Model file for the job. Use its own axes, mm. Give positions to 0.01 mm unless a question says otherwise; leave off trailing zeros. Order: outer loops, then holes, each group sorted by start corner. A loop starts at its lowest first (then second) coordinate and runs counter-clockwise, first axis right, second up. Notation, with made-up numbers: (40, -7.75) -> (70, -7.75) arc R20 ccw to (70, 24.25) -> close; hole circle Ø1 at (64.5, 18). An arc over 180 degrees is marked (long way). Use CSV: the item, a comma, the result in double quotes. Start each with the question number.
1. Cut at A-A on y = 92.5. List the corners of the cut face in (x, z).
2. Wall check: line 1 (Z direction, x = 8.5, y = 61); line 2 (X direction, y = -66.5, z = 1.75); line 3 (X direction, y = -39, z = 2). Give the ranges that are in metal, low to high. Write a range as from..to.
3. Cut at B-B on x = 42.5. List the corners of the cut face in (y, z), then the cut area to 3 significant figures.
4. Cut at D-D on y = -54. List the corners of the cut face in (x, z), then the cut area to 3 significant figures.
5. Drop flat-ended pins along their axis: pin 1 (4.5 mm diameter, centred on x = -48.94, y = -85.6, fed in from -Z); pin 2 (4.5 mm diameter, centred on x = 48.94, y = -85.6, fed in from +Z); pin 3 (8 mm diameter, centred on x = -41, z = -6, fed in from -Y). Give the stop position or say it passes through.
6. Cut at C-C on x = -9. List the corners of the cut face in (y, z).
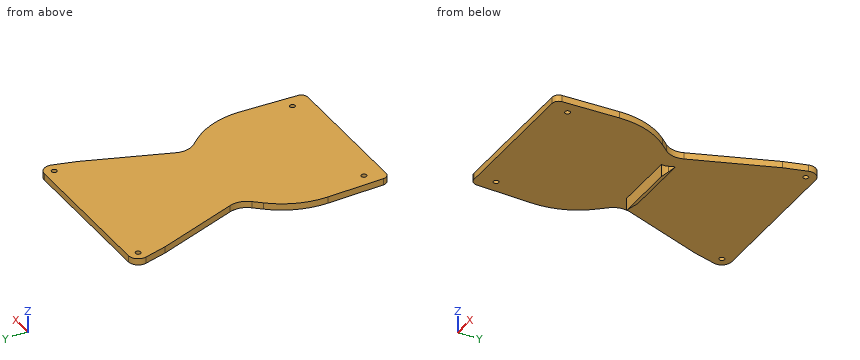
```python
from build123d import *

# Parameters (mm, degrees)
SKETCH1_R           = 2
BOSS_EXTRUDE1_DEPTH = 5
BOSS_EXTRUDE2_DEPTH = 10
CHAMFER2_SIZE       = 10


with BuildPart() as part:
    # Sketch1 → Boss-Extrude1 (new body)
    with BuildSketch(Plane.XY):
        with BuildLine():
            Line((-39.95406266, -4.540740277), (-45.172708428, -10.510426525))
            ThreePointArc((-45.172708428, -10.510426525), (-56.503917554, -29.818144261), (-59.968772691, -51.935536587))
            Line((-59.968772691, -51.935536587), (-58.57362931, -95.161294716))
            ThreePointArc((-58.57362931, -95.161294716), (-57.054271725, -98.592107569), (-53.576231585, -100))
            Line((-53.576231585, -100), (-50, -100))
            Line((-50, -100), (50, -100))
            Line((50, -100), (53.576231585, -100))
            ThreePointArc((53.576231585, -100), (57.054271725, -98.592107569), (58.57362931, -95.161294716))
            Line((58.57362931, -95.161294716), (59.968772691, -51.935536587))
            ThreePointArc((59.968772691, -51.935536587), (56.503917554, -29.818144261), (45.172708428, -10.510426525))
            Line((45.172708428, -10.510426525), (39.95406266, -4.540740277))
            ThreePointArc((39.95406266, -4.540740277), (36.502239109, 2.577573283), (37.151850455, 10.461955241))
            Line((37.151850455, 10.461955241), (60, 73.236730193))
            Line((60, 73.236730193), (64.733567494, 90.51871221))
            ThreePointArc((64.733567494, 90.51871221), (63.462787034, 97.049194521), (57.5, 100))
            Line((57.5, 100), (55, 100))
            Line((55, 100), (-55, 100))
            Line((-55, 100), (-57.5, 100))
            ThreePointArc((-57.5, 100), (-63.462787034, 97.049194521), (-64.733567494, 90.51871221))
            Line((-64.733567494, 90.51871221), (-60, 73.236730193))
            Line((-60, 73.236730193), (-37.151850455, 10.461955241))
            ThreePointArc((-37.151850455, 10.461955241), (-36.502239109, 2.577573283), (-39.95406266, -4.540740277))
        make_face()
        with Locations((-57.5, 92.5)):
            Circle(SKETCH1_R, mode=Mode.SUBTRACT)
        with Locations((57.5, 92.5)):
            Circle(SKETCH1_R, mode=Mode.SUBTRACT)
        with Locations((48.939097244, -85.598196118)):
            Circle(SKETCH1_R, mode=Mode.SUBTRACT)
        with Locations((-48.939097244, -85.598196118)):
            Circle(SKETCH1_R, mode=Mode.SUBTRACT)
    extrude(amount=BOSS_EXTRUDE1_DEPTH)

    # Sketch2 → Boss-Extrude2 (add)
    with BuildSketch(Plane(origin=(0, 0, 0), x_dir=(-1, 0, 0), z_dir=(0, 0, -1))):
        with BuildLine():
            Line((-23.747944524, 0.5), (23.747944524, 0.5))
            ThreePointArc((23.747944524, 0.5), (23.669056818, 3.144030102), (24.253462846, 5.723872742))
            Line((24.253462846, 5.723872742), (25.870507592, 10.166666667))
            Line((25.870507592, 10.166666667), (-25.870507592, 10.166666667))
            Line((-25.870507592, 10.166666667), (-24.253462846, 5.723872742))
            ThreePointArc((-24.253462846, 5.723872742), (-23.669056818, 3.144030102), (-23.747944524, 0.5))
        make_face()
    extrude(amount=BOSS_EXTRUDE2_DEPTH)

    # Chamfer2
    # the kernel refuses this chamfer: 10 mm, written as the material it takes off along each edge
    with BuildSketch(Plane(origin=(-51.587337472, 10.166666667, -10), x_dir=(0, 0.027495876610586317, 0.9996219169112968), z_dir=(1, 0, 0))) as chamfer2_piece_1_section:
        Polygon((CHAMFER2_SIZE * 0.999621916911, CHAMFER2_SIZE * 0.0274958766106), (-CHAMFER2_SIZE * 0.0274958766106, CHAMFER2_SIZE * 0.999621916911), (0, 0), align=None)
    chamfer2_piece_1 = extrude(amount=103.174674944, mode=Mode.PRIVATE)
    chamfer2_piece_1 = split(chamfer2_piece_1, bisect_by=Plane(origin=(0, 6.862625123, 0), z_dir=(0, 0, -1)), keep=Keep.TOP, mode=Mode.PRIVATE)
    add(chamfer2_piece_1, mode=Mode.SUBTRACT)


solid = part.part
```
Verdict:
1,outline,"(-65, 0) -> (-59.5, 0) -> (-59.5, 5) -> (-65, 5) -> close; (-55.5, 0) -> (55.5, 0) -> (55.5, 5) -> (-55.5, 5) -> close; (59.5, 0) -> (65, 0) -> (65, 5) -> (59.5, 5) -> close"
2,line 1,"0..5"
2,line 2,"-59.5..59.5"
2,line 3,"-58.98..58.98"
3,outline,"(-100, 0) -> (-7.45, 0) -> (-7.45, 5) -> (-100, 5) -> close; (25.16, 0) -> (100, 0) -> (100, 5) -> (25.16, 5) -> close"
3,area,"837 mm^2"
4,outline,"(-59.9, 0) -> (59.9, 0) -> (59.9, 5) -> (-59.9, 5) -> close"
4,area,"599 mm^2"
5,pin 1,"z = 0"
5,pin 2,"z = 5"
5,pin 3,"through"
6,outline,"(-100, 0) -> (0.5, 0) -> (0.5, -9.67) -> (10.17, 0) -> (100, 0) -> (100, 5) -> (-100, 5) -> close"
